For this review, take the finished solid that the model builds, in its own axes (mm). Face numbers are marked on the shaded views. A direction names the side the tool comes from. Round coordinates to 2 decimals unless told otherwise and drop trailing zeros. Order: outer loops, then holes, each group sorted by start corner. A loop starts at its lowest first (then second) coordinate and runs counter-clockwise, first axis right, second up. Notation, with made-up numbers: (6.25, 71.5) - (37.25, 71.5) arc R32 cw to (37.25, 99.5) - close; hole circle Ø1 at (-9, 80). An arc over 180 degrees is marked (long way). One line per item, written item: value.
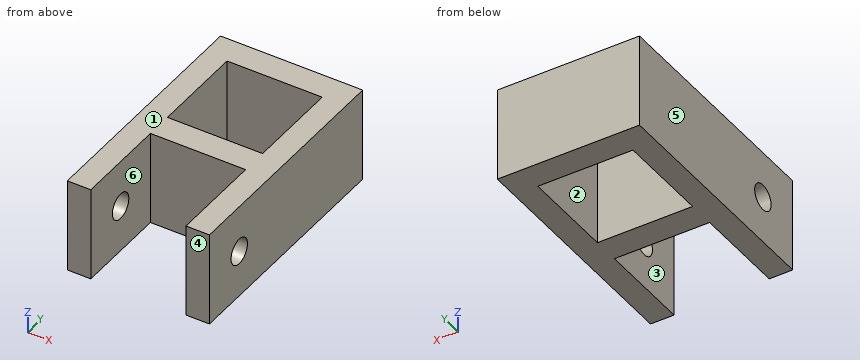
```python
from build123d import *

# Parameters (mm, degrees)
SKETCH1_W               = 20.25
SKETCH1_H               = 20
BOSS_EXTRUDE1_DEPTH     = 20
CUT_EXTRUDE1_DEPTH      = 58.19025813
CUT_EXTRUDE1_DEPTH_BACK = 58.19025813
SKETCH2_R               = 2.75


with BuildPart() as part:
    # Sketch1 → Boss-Extrude1 (new body)
    with BuildSketch(Plane.XY):
        Polygon((-10.125, 0), (-10.125, 20), (10.125, 20), (10.125, 0), (15.125, 0), (15.125, 51.4), (-15.125, 51.4), (-15.125, 0), align=None)
        with Locations((0, 35.7)):
            Rectangle(SKETCH1_W, SKETCH1_H, mode=Mode.SUBTRACT)
    extrude(amount=BOSS_EXTRUDE1_DEPTH)

    # Sketch2 → Cut-Extrude1 (cut, two sides: drawn at the far end of the back side and taken through both)
    with BuildSketch(Plane(origin=(0, 0, 0), x_dir=(0, 0, -1), z_dir=(1, 0, 0)).offset(-CUT_EXTRUDE1_DEPTH_BACK)):
        with Locations((-10, 10)):
            Circle(SKETCH2_R)
    extrude(amount=CUT_EXTRUDE1_DEPTH + CUT_EXTRUDE1_DEPTH_BACK, mode=Mode.SUBTRACT)


solid = part.part
```
Item 1: The part is to be moulded in two halves that separate along X. For the marked faces 4, 5 and 6, say which applies: +X half, -X half, draft (parallel to the pull), parting line (faces both ways), or undercut.
Returned:
face 4: draft
face 5: -X half
face 6: undercut
Item 2: Take a section at C-C (z = 10). Write out the cut boundary in (x, y) (3 decimals).
Returned:
outline: (-15.125, 0) - (-10.125, 0) - (-10.125, 7.25) - (-15.125, 7.25) - close; (-15.125, 12.75) - (-10.125, 12.75) - (-10.125, 20) - (10.125, 20) - (10.125, 12.75) - (15.125, 12.75) - (15.125, 51.4) - (-15.125, 51.4) - close; (10.125, 0) - (15.125, 0) - (15.125, 7.25) - (10.125, 7.25) - close; hole (-10.125, 25.7) - (10.125, 25.7) - (10.125, 45.7) - (-10.125, 45.7) - close
Item 3: For P1, Ø10, axis at x = 0.5, z = 6.5, coming from the -Y side; P2, Ø12, axis at x = -3, y = 7.5, coming from the -Z side, all flat-tipped, find the tip position at first contact; note any pin that passes through.
Returned:
P1: y = 20
P2: through
Item 4: Wall thickness on line 1 (Z direction, x = 14, y = 10); line 2 (Y direction, x = -7.5, z = 8.5); line 3 (X direction, y = 6, z = 18.5) (3 decimals): over which ranges is each line inside the solid? List them lowest first.
Returned:
line 1: 0 to 7.25, 12.75 to 20
line 2: 20 to 25.7, 45.7 to 51.4
line 3: -15.125 to -10.125, 10.125 to 15.125
Item 5: Machinability: for the marked faces 1, 2 and 3, which of the approach directions +Z, -Z, +X, -X, +Y, -Y give a long, thin tool a straight path to every point of the face, cutting with its end or side? Answer none if there is none.
Returned:
face 1: +Z, +X, -X, +Y, -Y
face 2: +Z, -Z
face 3: +Z, -Z, -Y
Item 6: Take a section at B-B (y = 18). Write out the cut boundary in (x, z) (3 decimals), plus the area to 3 significant figures.
Returned:
outline: (-15.125, 0) - (-10.125, 0) - (-10.125, 20) - (-15.125, 20) - close; (10.125, 0) - (15.125, 0) - (15.125, 20) - (10.125, 20) - close
area: 200 mm^2
Item 7: Take a section at A-A (x = -9). Write out the cut boundary in (y, z).
Returned:
outline: (20, 0) - (25.7, 0) - (25.7, 20) - (20, 20) - close; (45.7, 0) - (51.4, 0) - (51.4, 20) - (45.7, 20) - close
Item 8: Take a section at D-D (z = 2.25). Write out the cut boundary in (x, y) (3 decimals).
Returned:
outline: (-15.125, 0) - (-10.125, 0) - (-10.125, 20) - (10.125, 20) - (10.125, 0) - (15.125, 0) - (15.125, 51.4) - (-15.125, 51.4) - close; hole (-10.125, 25.7) - (10.125, 25.7) - (10.125, 45.7) - (-10.125, 45.7) - close
